from build123d import *

# Parameters (mm, degrees)
BOSS_EXTRUDE1_DEPTH    = 6.35
F_10_32_TAPPED_HOLE1_D = 4.0386
F_10_32_TAPPED_HOLE2_D = 4.0386
F_6_CLEARANCE_HOLE1_D  = 3.7973


with BuildPart() as part:
    # Sketch1 → Boss-Extrude1 (new body)
    with BuildSketch(Plane.XY):
        Polygon((-35.6340909, 17.237993597), (-15.089584497, 37.7825), (-12.7, 37.7825), (-12.7, 63.1825), (12.7, 63.1825), (12.7, 37.7825), (15.089584497, 37.7825), (37.865937227, 15.00614727), (37.865937227, -16.815626239), (16.105313466, -38.57625), (-3.96875, -38.57625), (-3.96875, -30.95625), (12.949006121, -30.95625), (30.245937227, -13.659318894), (30.245937227, 11.849839924), (11.933277152, 30.1625), (-11.933277152, 30.1625), (-30.245937227, 11.849839924), align=None)
    extrude(amount=BOSS_EXTRUDE1_DEPTH)

    # #10-32 Tapped Hole1 (through all)
    with Locations(Plane.XY.offset(6.35)):
        with Locations((-30.245937227, 16.339967985)):
            Hole(F_10_32_TAPPED_HOLE1_D / 2)

    # #10-32 Tapped Hole2 (through all)
    with Locations(Plane.XY.offset(6.35)):
        with Locations((30.245937227, 16.339967985), (-0.79375, -34.13125)):
            Hole(F_10_32_TAPPED_HOLE2_D / 2)

    # #6 Clearance Hole1 (through all)
    with Locations(Plane(origin=(-6.35, 56.8325, 6.35), x_dir=(1, 0, 0), z_dir=(0, 0, 1))):
        with Locations((0, 0), (12.7, 0)):
            Hole(F_6_CLEARANCE_HOLE1_D / 2)


solid = part.part
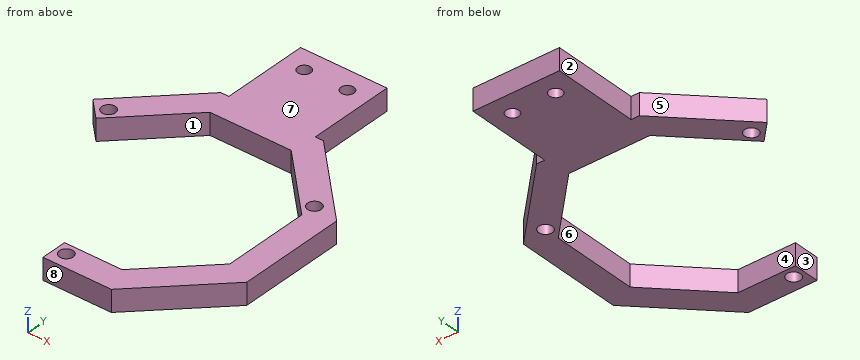
Check sheet for the modelled part. Datum: model origin and axes. Units: mm. Face numbers are marked on the shaded views. A direction names the side the tool comes from. Coordinates: 2 decimals unless noted, no trailing zeros. Write each loop counter-clockwise with the first axis right and the second up, starting at its lowest first coordinate (ties: lowest second). Pieces come first, ordered by that corner, then holes. Notation, with made-up numbers: M 3.5,5 L 39.5,5 A13 cw 39.5,20 Z; hole C 52.25,28 d3. An arc over 180 degrees is marked long. Answer as CSV lines item,"result".
Q1. Material ranges on probe 1 along Y at (x, z) = (-6.35, 4.5); probe 2 along X at (y, z) = (-13.5, 2.75); probe 3 along Y at (x, z) = (2, 3.75), recorded low to high. Write a range as from..to.
Check result:
probe 1,"30.16..54.93, 58.73..63.18"
probe 2,"30.25..37.87"
probe 3,"-38.58..-30.96, 30.16..63.18"
Q2. Cross-section at C-C (z = 3.75). Record the boundary of the cut face in (x, y).
Check result:
outline,"M -35.63,17.24 L -30.25,11.85 L -11.93,30.16 L 11.93,30.16 L 30.25,11.85 L 30.25,-13.66 L 12.95,-30.96 L -3.97,-30.96 L -3.97,-38.58 L 16.11,-38.58 L 37.87,-16.82 L 37.87,15.01 L 15.09,37.78 L 12.7,37.78 L 12.7,63.18 L -12.7,63.18 L -12.7,37.78 L -15.09,37.78 Z; hole C -30.25,16.34 d4.04; hole C -6.35,56.83 d3.8; hole C -0.79,-34.13 d4.04; hole C 6.35,56.83 d3.8; hole C 30.25,16.34 d4.04"
Q3. Go/stop test with flat-tipped pins: pin 1 (2 mm diameter, centred on y = 5, z = 1.5, fed in from -X); pin 2 (3 mm diameter, centred on y = 49, z = 3.5, fed in from +X); pin 3 (1.9 mm diameter, centred on x = -14, z = 3, fed in from +Y). Record where each tip stops, or that it passes through.
Check result:
pin 1,"x = 30.25"
pin 2,"x = 12.7"
pin 3,"y = 37.78"
Q4. Cross-section at B-B (y = 25). Record the boundary of the cut face in (x, z), then the cut area to 3 significant figures.
Check result:
outline,"M -27.87,0 L -17.1,0 L -17.1,6.35 L -27.87,6.35 Z; M 17.1,0 L 27.87,0 L 27.87,6.35 L 17.1,6.35 Z"
area,"137 mm^2"
Q5. Cross-section at A-A (x = 9.5). Record the boundary of the cut face in (y, z), then the cut area to 3 significant figures.
Check result:
outline,"M -38.58,0 L -30.96,0 L -30.96,6.35 L -38.58,6.35 Z; M 30.16,0 L 63.18,0 L 63.18,6.35 L 30.16,6.35 Z"
area,"258 mm^2"
Q6. Cross-section at D-D (y = 0). Record the boundary of the cut face in (x, z).
Check result:
outline,"M 30.25,0 L 37.87,0 L 37.87,6.35 L 30.25,6.35 Z"
Q7. Set-up check for the marked faces 1, 2, 3 and 4: record each of +Z, -Z, +X, -X, +Y, -Y from which the full face is reachable in a straight line by a thin tool's end or side.
Check result:
face 1,"+Z, -Z, -Y"
face 2,"+Z, -Z, -X, +Y"
face 3,"+Z, -Z, -X, -Y"
face 4,"+Z, -Z, -X"
Q8. Mould release check, pull along Y, two halves, no side actions. Record for the marked faces 5, 6, 7 and 8: released by +Y, released by -Y, zero draft, split by the parting line, or undercut.
Check result:
face 5,"released by +Y"
face 6,"undercut"
face 7,"zero draft"
face 8,"released by -Y"
